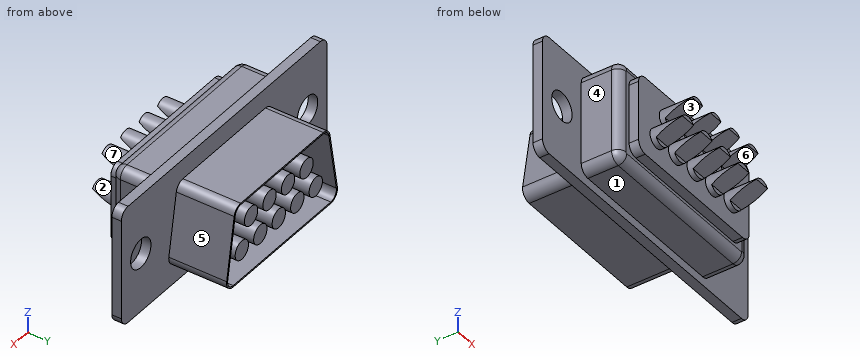
Autodesk Inventor part; units mm, degrees
ref_plane "YZ Plane" through (0, 0, 0) normal (1, 0, 0) x (0, 1, 0)
ref_plane "XZ Plane" through (0, 0, 0) normal (0, 1, 0) x (-1, 0, 0)
ref_plane "XY Plane" through (0, 0, 0) normal (0, 0, 1) x (1, 0, 0)
sketch "Sketch1" plane through (0, 0, 0) normal (0, 1, 0) x (-1, 0, 0)
  line L0 (-14.405, 6.275) -> (14.405, 6.275)
  line L1 (15.405, 5.275) -> (15.405, -5.275)
  line L2 (14.405, -6.275) -> (-14.405, -6.275)
  line L3 (-15.405, -5.275) -> (-15.405, 5.275)
  arc A0 (-14.405, 6.275) -> (-15.405, 5.275) centre (-14.405, 5.275) ccw
  arc A1 (15.405, 5.275) -> (14.405, 6.275) centre (14.405, 5.275) ccw
  arc A2 (14.405, -6.275) -> (15.405, -5.275) centre (14.405, -5.275) ccw
  arc A3 (-15.405, -5.275) -> (-14.405, -6.275) centre (-14.405, -5.275) ccw
  circle A4 centre (12.495, 0) radius 1.525
  circle A5 centre (-12.495, 0) radius 1.525
  point P0 (0, 0)
  point P1 (-15.405, 6.275)
  point P2 (15.405, -6.275)
  point P3 (15.405, 6.275)
  dimension "d0" = 30.81
  dimension "d1" = 12.55
  dimension "d2" = 6.275
  dimension "d3" = 15.405
  dimension "d4" = 1
  dimension "d16" = 3.05
  dimension "d17" = 3.05
  dimension "d18" = 24.99
  dimension "d19" = 12.495
extrude "Extrusion1" add sketch "Sketch1" along normal blind 1
sketch "Sketch2" plane through (0, 1, 0) normal (0, 1, 0) x (1, 0, 0)
  line L0 (-7.3082, 4.18) -> (7.3082, 4.18)
  line L1 (8.5, 4.18) -> (8.5, -4.18)
  line L2 (6.1868, -4.18) -> (-6.1868, -4.18)
  line L3 (-8.5, -4.18) -> (-8.5, 4.18)
  line L4 (-8.2931, 3.0064) -> (-7.1716, -3.3536)
  line L5 (8.2931, 3.0064) -> (7.1716, -3.3536)
  arc A0 (-7.3082, 4.18) -> (-8.2931, 3.0064) centre (-7.3082, 3.18) ccw
  arc A1 (-7.1716, -3.3536) -> (-6.1868, -4.18) centre (-6.1868, -3.18) ccw
  arc A2 (6.1868, -4.18) -> (7.1716, -3.3536) centre (6.1868, -3.18) ccw
  arc A3 (8.2931, 3.0064) -> (7.3082, 4.18) centre (7.3082, 3.18) ccw
  line L6 (7.3082, 4.0255) -> (-7.3082, 4.0255)
  arc A4 (-7.3082, 4.0255) -> (-8.1409, 3.0332) centre (-7.3082, 3.18) ccw
  line L7 (-8.1409, 3.0332) -> (-7.0195, -3.3268)
  arc A5 (-7.0195, -3.3268) -> (-6.1868, -4.0255) centre (-6.1868, -3.18) ccw
  line L8 (-6.1868, -4.0255) -> (6.1868, -4.0255)
  arc A6 (6.1868, -4.0255) -> (7.0195, -3.3268) centre (6.1868, -3.18) ccw
  line L9 (7.0195, -3.3268) -> (8.1409, 3.0332)
  arc A7 (8.1409, 3.0332) -> (7.3082, 4.0255) centre (7.3082, 3.18) ccw
  point P0 (0, 0)
  dimension "d7" = 17
  dimension "d8" = 8.36
  dimension "d9" = 4.18
  dimension "d10" = 8.5
  dimension "d11" = 10
  dimension "d12" = 10
  dimension "d13" = 1
extrude "Extrusion2" add sketch "Sketch2" along normal blind 6.1
sketch "Sketch3" plane through (0, 0, 0) normal (0, -1, 0) x (1, 0, 0)
  line L0 (-8.6, 5.36) -> (8.6, 5.36)
  line L1 (9.6, 4.36) -> (9.6, -4.36)
  line L2 (8.6, -5.36) -> (-8.6, -5.36)
  line L3 (-9.6, -4.36) -> (-9.6, 4.36)
  arc A0 (-8.6, 5.36) -> (-9.6, 4.36) centre (-8.6, 4.36) ccw
  arc A1 (9.6, 4.36) -> (8.6, 5.36) centre (8.6, 4.36) ccw
  arc A2 (8.6, -5.36) -> (9.6, -4.36) centre (8.6, -4.36) ccw
  arc A3 (-9.6, -4.36) -> (-8.6, -5.36) centre (-8.6, -4.36) ccw
  point P0 (0, 0)
  point P1 (-9.6, 5.36)
  point P2 (9.6, -5.36)
  point P3 (9.6, 5.36)
  dimension "d20" = 19.2
  dimension "d21" = 10.72
  dimension "d22" = 5.36
  dimension "d23" = 9.6
  dimension "d24" = 1
extrude "Extrusion3" add sketch "Sketch3" along normal blind 4.1
fillet "Fillet1" radius 0.9 8 edges at (9.3071, -4.1, -5.0671) (9.6, -4.1, 0) (9.3071, -4.1, 5.0671) (0, -4.1, 5.36) (-9.3071, -4.1, 5.0671) (-9.6, -4.1, 0) (-9.3071, -4.1, -5.0671) (0, -4.1, -5.36)
sketch "Sketch4" plane through (0, -4.1, 0) normal (0, -1, 0) x (1, 0, 0)
  line L0 (-7.2476, 4.1431) -> (7.3248, 4.1431)
  line L1 (8.3248, 3.1431) -> (8.3248, -3.1174)
  line L2 (7.3248, -4.1174) -> (-7.2476, -4.1174)
  line L3 (-8.2476, -3.1174) -> (-8.2476, 3.1431)
  arc A0 (-7.2476, 4.1431) -> (-8.2476, 3.1431) centre (-7.2476, 3.1431) ccw
  arc A1 (8.3248, 3.1431) -> (7.3248, 4.1431) centre (7.3248, 3.1431) ccw
  arc A2 (7.3248, -4.1174) -> (8.3248, -3.1174) centre (7.3248, -3.1174) ccw
  arc A3 (-8.2476, -3.1174) -> (-7.2476, -4.1174) centre (-7.2476, -3.1174) ccw
  point P0 (0, 0)
  point P1 (-8.2476, 4.1431)
  point P2 (8.3248, -4.1174)
  point P3 (8.3248, 4.1431)
  point P4 (-8.2476, -4.1174)
  dimension "d30" = 1
extrude "Extrusion4" add sketch "Sketch4" along normal blind 1
sketch "Sketch5" plane through (0, 1, 0) normal (0, 1, 0) x (1, 0, 0)
  line L0 (7.3082, 4.0255) -> (-7.3082, 4.0255)
  circle A0 centre (-5.54, 1.42) radius 1
  circle A1 centre (-4.155, -1.42) radius 1
  circle A2 centre (-2.77, 1.42) radius 1
  circle A3 centre (0, 1.42) radius 1
  circle A4 centre (2.77, 1.42) radius 1
  circle A5 centre (5.54, 1.42) radius 1
  circle A6 centre (-1.385, -1.42) radius 1
  circle A7 centre (1.385, -1.42) radius 1
  circle A8 centre (4.155, -1.42) radius 1
  point P0 (0, 0)
  dimension "d31" = 5.54
  dimension "d32" = 4.155
  dimension "d34" = 1.42
  dimension "d35" = 1.42
  dimension "d36" = 2
  dimension "d37" = 2
  dimension "d40" = 2.77
  dimension "d47" = 2.77
extrude "Extrusion5" add sketch "Sketch5" along normal blind 5.7625 and the other way blind 9.4
sketch "Sketch6" plane through (-9.6, 0, -4.36) normal (-1, 0, 0) x (0, 0, 1)
  line L0 (0, 0) -> (0, -3.2)
  line L1 (1.538, -5.6397) -> (2.3945, -5.6397)
  line L2 (2.3945, -5.6397) -> (3.6462, -8.7799)
  line L3 (3.6462, -8.7799) -> (1.538, -8.7799)
  line L4 (1.538, -8.7799) -> (1.538, -5.6397)
  line L5 (4.4367, -5.6397) -> (5.2932, -5.6397)
  line L6 (5.2932, -5.6397) -> (6.5449, -8.7799)
  line L7 (6.5449, -8.7799) -> (4.4367, -8.7799)
  line L8 (4.4367, -8.7799) -> (4.4367, -5.6397)
  point P0 (4.36, 0)
extrude "Extrusion6" cut sketch "Sketch6" against normal through all
properties part number "DSUB_9_Male"
Verification items for the finished model (mm, model axes). Face numbers are marked on the shaded views. A direction names the side the tool comes from. Give positions to 0.01 mm unless a question says otherwise; leave off trailing zeros.
1. Mould release check, pull along X, two halves, no side actions. Record for the marked faces 4, 5, 6 and 7: released by +X, released by -X, zero draft, split by the parting line, or undercut.
2. Thickness scan on line 1 (Z direction, x = -1.5, y = 3.5); line 2 (Z direction, x = 2, y = 4.5); line 3 (Z direction, x = 5, y = -2.5). Record the ranges inside material, lowest first.
3. Set-up check for the marked faces 1, 2 and 3: record each of +Z, -Z, +X, -X, +Y, -Y from which the full face is reachable in a straight line by a thin tool's end or side.
4. Section check A-A, the plane y = 2.5. Count the separate pieces of the cut face and the enclosed holes in it, then the cut area to 3 significant figures.
5. Go/stop test with flat-tipped pins: pin 1 Ø3 at (x, y) = (-0.5, 3.5) entering from -Z; pin 2 Ø3 at (x, y) = (3, 4) entering from +Z; pin 3 Ø3 at (x, y) = (2, -2.5) entering from -Z. Record where each tip stops, or that it passes through.
Geometry says:
1. face 4: released by -X
1. face 5: released by +X
1. face 6: zero draft
1. face 7: undercut
2. line 1: z = -4.18 to -4.03, 0.43 to 2.41, 4.03 to 4.18
2. line 2: z = -4.18 to -4.03, -2.06 to -0.78, 0.63 to 2.21, 4.03 to 4.18
2. line 3: z = -5.36 to 5.36
3. face 1: -Z, +X, -X, -Y
3. face 2: -Y
3. face 3: +X, -X, -Y
4. separate pieces: 10
4. enclosed holes: 1
4. area: 35.3 mm2
5. pin 1: stops at z = -4.18
5. pin 2: stops at z = 4.18
5. pin 3: stops at z = -5.36
